Answer from the drawing. Dimensions are ordinates in mm from the lowest x, y and z of the part. A direction names the side the tool comes from. Round coordinates to 2 decimals unless told otherwise and drop trailing zeros. Loops run counter-clockwise (first coordinate to the right, second up) from the corner with the lowest first, then second, coordinate; pieces in that order, holes last. Notation, with made-up numbers: (86.25, 59.5) - (100.25, 59.5) arc R13 cw to (100.25, 74.5) - close; hole circle Ø4 at (73.5, 41). An arc over 180 degrees is marked (long way). Answer as CSV lines item,"result". Start each with the question number.
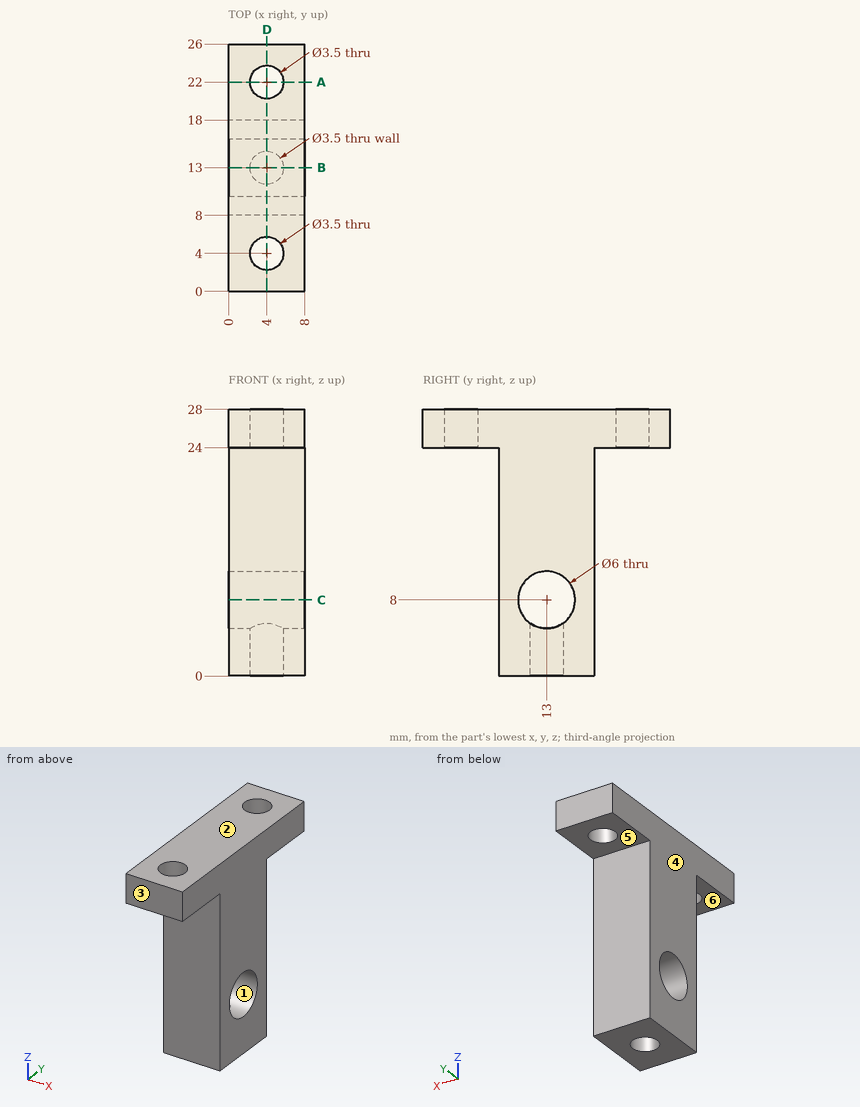
Item 1: Section A-A, the plane y = 22 is taken. Give the vertices of the cut face in (x, z).
Item 2: Section B-B, the plane y = 13 is taken. Give the vertices of the cut face in (x, z).
Item 3: Section C-C, the plane z = 8 is taken. Give the vertices of the cut face in (x, y).
Item 4: Find the intervals of material crossed by L1, parallel to Y at x = 4, z = 25.25; L2, parallel to Y at x = 4, z = 3.25; L3, parallel to X at y = 13, z = 3.75, in increasing order.
Item 5: Determine the mould class of the marked faces 1, 2 and 3 for opening direction Z: pulls with the +Z half, pulls with the -Z half, needs draft (parallel to the pull), parting line crosses it, or undercut.
Item 6: Which of the six approach directions +Z, -Z, +X, -X, +Y, -Y give full straight-line access (tool end or side, diameter ignored) to the marked faces 4, 5 and 6?
Item 7: Flat-ended cylindrical pins translate along their axes: pin 1 Ø3 at (x, y) = (4, 22) entering from -Z; pin 2 Ø2.5 at (x, z) = (3.5, 12) entering from -Y; pin 3 Ø1 at (x, z) = (5.5, 18) entering from +Y. Find the tip coordinate at first contact, or state that the pin passes through.
Item 8: Section D-D, the plane x = 4 is taken. Give the vertices of the cut face in (y, z).
Answer:
1,outline,"(0, 24) - (2.25, 24) - (2.25, 28) - (0, 28) - close; (5.75, 24) - (8, 24) - (8, 28) - (5.75, 28) - close"
2,outline,"(0, 0) - (2.25, 0) - (2.25, 5) - (0, 5) - close; (0, 11) - (8, 11) - (8, 28) - (0, 28) - close; (5.75, 0) - (8, 0) - (8, 5) - (5.75, 5) - close"
3,outline,"(0, 8) - (8, 8) - (8, 10) - (0, 10) - close; (0, 16) - (8, 16) - (8, 18) - (0, 18) - close"
4,L1,"y = 0 to 2.25, 5.75 to 20.25, 23.75 to 26"
4,L2,"y = 8 to 11.25, 14.75 to 18"
4,L3,"x = 0 to 2.25, 5.75 to 8"
5,face 1,"undercut"
5,face 2,"pulls with the +Z half"
5,face 3,"needs draft"
6,face 4,"+Z, -Z, -X, +Y, -Y"
6,face 5,"-Z, +X, -X, +Y"
6,face 6,"-Z, +X, -X, -Y"
7,pin 1,"passes through"
7,pin 2,"stops at y = 8"
7,pin 3,"stops at y = 18"
8,outline,"(0, 24) - (2.25, 24) - (2.25, 28) - (0, 28) - close; (5.75, 24) - (8, 24) - (8, 0) - (11.25, 0) - (11.25, 5.56) arc R3 cw (long way) to (14.75, 5.56) - (14.75, 0) - (18, 0) - (18, 24) - (20.25, 24) - (20.25, 28) - (5.75, 28) - close; (23.75, 24) - (26, 24) - (26, 28) - (23.75, 28) - close"
